Input: part model. Units: mm. Frame: model coordinates. Face numbers are marked on the shaded views. A direction names the side the tool comes from. Coordinates: 2 decimals unless noted, no trailing zeros. Loops run counter-clockwise (first coordinate to the right, second up) from the corner with the lowest first, then second, coordinate; pieces in that order, holes last. Notation, with made-up numbers: (41, -9) - (98, -9) arc R25 ccw to (98, 8) - close; hole circle Ø10 at (-21, -21.75). An arc over 180 degrees is marked (long way). Use a Markdown table: item, result. Add a question column.
1. Section query C-C on y = 24. Return the cut outline in (x, z), then the cut area to 3 significant figures.
2. Ray query, L1, parallel to Y at x = 55, z = 65.5; L2, parallel to X at y = 55.5, z = 58; L3, parallel to Z at x = 34, y = 61. Return the intervals inside material, ascending. Write a range as [from, to].
3. Section query D-D on x = 60. Return the cut outline in (y, z).
4. Section query B-B on x = 39. Return the cut outline in (y, z), then the cut area to 3 significant figures.
5. Draft query along Y for the marked faces 1, 2 and 3. Return one class per face: released by +Y, released by -Y, zero draft, split by the parting line, or undercut.
6. Section query A-A on z = 63.5. Return the cut outline in (x, y), then the cut area to 3 significant figures.
7. Contact query for a flat-ended pin moving along its axis: P1, Ø0.5, axis at x = 56, y = 62, coming from the +Z side. Output: stop coordinate, or through.
8. Access query for the marked faces 4 and 5. Directions: +Z, -Z, +X, -X, +Y, -Y. A direction counts if a zero-diameter tool reaches every point of the face in a straight line with its end or side. Return the directions, or none.
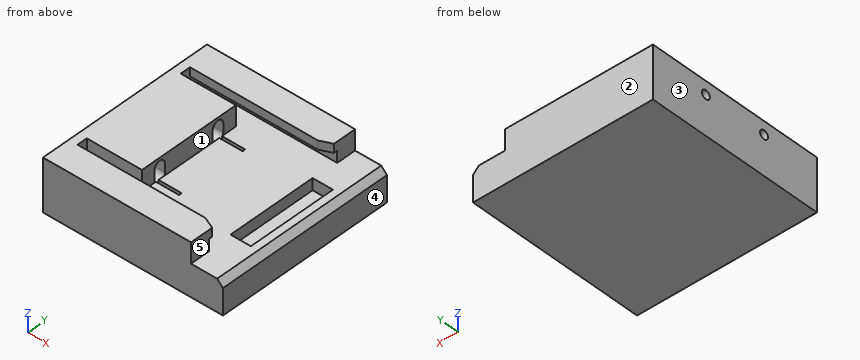
```python
from build123d import *

# Parameters (mm, degrees)
SKETCH072_W             = 62
SKETCH072_H             = 62
PAD012_DEPTH            = 18
POCKET059_DEPTH         = 59
POCKET060_DEPTH         = 7
SKETCH077_R             = 1.5
POCKET062_DEPTH         = 22
POCKET067_DEPTH         = 10
SKETCH076_W             = 31
SKETCH076_H             = 7
SKETCH076_W_2           = 1
SKETCH076_H_2           = 8
POCKET065_DEPTH         = 11
POCKET066_DEPTH         = 62.001
BODY012_PLACEMENT_ANGLE = 90


with BuildPart() as part:
    # Sketch072 → Pad012 (new body)
    with BuildSketch(Plane.XY):
        Rectangle(SKETCH072_W, SKETCH072_H)
    extrude(amount=PAD012_DEPTH)

    # Sketch074 → Pocket059 (cut)
    with BuildSketch(Plane.XZ.offset(31)):
        Polygon((-21.25, 20), (-21.25, 15), (-24.25, 15), (-24.25, 11), (-17.75, 11), (-17.75, 18), (17.75, 18), (17.75, 11), (24.25, 11), (24.25, 15), (21.25, 15), (21.25, 20), align=None)
    extrude(amount=-POCKET059_DEPTH, mode=Mode.SUBTRACT)

    # Sketch075 (on Face5 of Pocket059) → Pocket060 (cut)
    with BuildSketch(Plane.XY.offset(18)):
        Polygon((-19, -11), (-19, 9), (19, 9), (19, -11), (23, -20), (31, -20), (31, -31), (-31, -31), (-31, -20), (-23, -20), align=None)
    extrude(amount=-POCKET060_DEPTH, mode=Mode.SUBTRACT)

    # Sketch077 → Pocket062 (cut)
    with BuildSketch(Plane(origin=(0, 31, 0), x_dir=(-1, 0, 0), z_dir=(0, 1, 0))):
        with Locations((-11, 13.5)):
            Circle(SKETCH077_R)
        with Locations((11, 13.5)):
            Circle(SKETCH077_R)
    extrude(amount=-POCKET062_DEPTH, mode=Mode.SUBTRACT)

    # Sketch081 (on Face35 of Pocket062) → Pocket067 (cut)
    with BuildSketch(Plane.XZ.offset(-9)):
        with BuildLine():
            ThreePointArc((-9, 15), (-11, 17), (-13, 15))
            Line((-13, 15), (-13, 12))
            ThreePointArc((-13, 12), (-11, 10), (-9, 12))
            Line((-9, 15), (-9, 12))
        make_face()
        with BuildLine():
            ThreePointArc((13, 15), (11, 17), (9, 15))
            Line((9, 15), (9, 12))
            ThreePointArc((9, 12), (11, 10), (13, 12))
            Line((13, 15), (13, 12))
        make_face()
    extrude(amount=-POCKET067_DEPTH, mode=Mode.SUBTRACT)

    # Sketch076 (on Face4 of Pocket060) → Pocket065 (cut)
    with BuildSketch(Plane.XY.offset(18)):
        with Locations((0, -23)):
            Rectangle(SKETCH076_W, SKETCH076_H)
        with Locations((-12, 5)):
            Rectangle(SKETCH076_W_2, SKETCH076_H_2)
        with Locations((12, 5)):
            Rectangle(SKETCH076_W_2, SKETCH076_H_2)
    extrude(amount=-POCKET065_DEPTH, mode=Mode.SUBTRACT)

    # Sketch080 (on Face8 of Pocket065) → Pocket066 (cut, through all)
    with BuildSketch(Plane.YZ.offset(31)):
        Polygon((-31, 11), (-31, 9), (-29, 11), align=None)
    extrude(amount=-POCKET066_DEPTH, mode=Mode.SUBTRACT)


with BuildPart() as part_1:
    # Body012 placement: moved
    add(part.part.moved(Location((60, 50, 50))).rotate(Axis((60, 50, 50), (0, 0, 1)), BODY012_PLACEMENT_ANGLE))


solid = part_1.part
```
Resolved:
| question | item | result |
|---|---|---|
| 1 | outline | (29, 50) - (91, 50) - (91, 59) - (89, 61) - (80, 61) - (80, 68) - (29, 68) - close |
| 1 | area | 1,040 mm² |
| 2 | L1 | [19, 28.75], [71.25, 81] |
| 2 | L2 | [29, 79.5], [86.5, 91] |
| 2 | L3 | [50, 62], [65, 68] |
| 3 | outline | (19, 50) - (81, 50) - (81, 68) - (71.25, 68) - (71.25, 65) - (74.25, 65) - (74.25, 61) - (25.75, 61) - (25.75, 65) - (28.75, 65) - (28.75, 68) - (19, 68) - close |
| 4 | outline | (19, 50) - (81, 50) - (81, 68) - (71.25, 68) - (71.25, 65) - (74.25, 65) - (74.25, 61) - (67.75, 61) - (67.75, 68) - (32.25, 68) - (32.25, 61) - (25.75, 61) - (25.75, 65) - (28.75, 65) - (28.75, 68) - (19, 68) - close; hole circle Ø3 at (39, 63.5); hole circle Ø3 at (61, 63.5) |
| 4 | area | 1,030 mm² |
| 5 | face 1 | undercut |
| 5 | face 2 | released by +Y |
| 5 | face 3 | zero draft |
| 6 | outline | (29, 19) - (80, 19) - (80, 25.75) - (32, 25.75) - (32, 32.25) - (51, 32.25) - (51, 37) - (41, 37) - (41, 37.5) - (29, 37.5) - close; (29, 40.5) - (41, 40.5) - (41, 41) - (51, 41) - (51, 59) - (41, 59) - (41, 59.5) - (29, 59.5) - close; (29, 62.5) - (41, 62.5) - (41, 63) - (51, 63) - (51, 67.75) - (32, 67.75) - (32, 74.25) - (80, 74.25) - (80, 81) - (29, 81) - close |
| 6 | area | 1,360 mm² |
| 7 | P1 | z = 57 |
| 8 | face 4 | +Z, -Z, +X, +Y, -Y |
| 8 | face 5 | +Z, +X, +Y, -Y |
